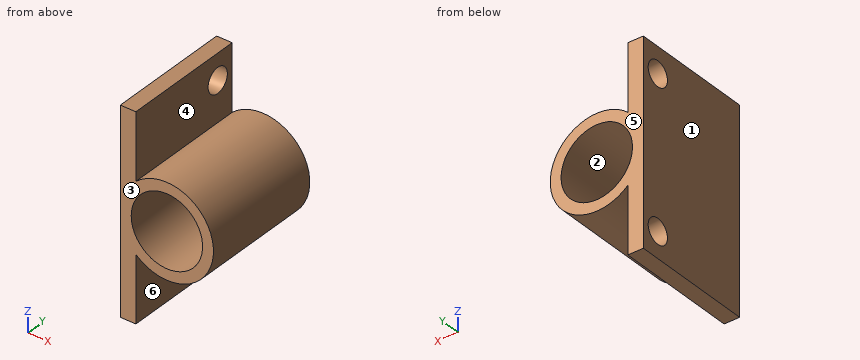
Autodesk Inventor part; units mm, degrees
ref_plane "YZ Plane" through (0, 0, 0) normal (1, 0, 0) x (0, 1, 0)
ref_plane "XZ Plane" through (0, 0, 0) normal (0, 1, 0) x (-1, 0, 0)
ref_plane "XY Plane" through (0, 0, 0) normal (0, 0, 1) x (1, 0, 0)
sketch "Sketch1" plane through (0, 0, 0) normal (0, 1, 0) x (-1, 0, 0)
  circle A0 centre (0, 0) radius 4.6
  line L0 (6, 13) -> (4, 13)
  line L1 (6, -13) -> (4, -13)
  arc A1 (4, 4.4721) -> (4, -4.4721) centre (0, 0) ccw
  line L2 (4, 13) -> (4, 4.4721)
  line L3 (4, -4.4721) -> (4, -13)
  line L4 (6, 13) -> (6, -13)
  dimension "d0" = 9.2
  dimension "d2" = 26
  dimension "d3" = 2
extrude "Extrusion1" add sketch "Sketch1" along normal blind 16
sketch "Sketch2" plane through (-6, 0, -13) normal (-1, 0, 0) x (0, 0, 1)
  circle A0 centre (3.35, 13.6) radius 1.6
  circle A1 centre (22.65, 13.6) radius 1.6
  line L0 (8.5279, 16) -> (0, 16)
  line L1 (0, 16) -> (26, 16)
  point P0 (13, 0)
  dimension "d10" = 3.2
  dimension "d11" = 3.2
  dimension "d14" = 2.4
  dimension "d15" = 2.4
extrude "Extrusion2" cut sketch "Sketch2" against normal blind 16
properties part number "Support endStop v2"
Geometry: final body of the model. Coordinates: model frame, mm. Face numbers are marked on the shaded views. A direction names the side the tool comes from. Round coordinates to 2 decimals unless told otherwise and drop trailing zeros. Loops run counter-clockwise (first coordinate to the right, second up) from the corner with the lowest first, then second, coordinate; pieces in that order, holes last. Notation, with made-up numbers: M -35.75,20.5 L 5.25,20.5 A26 ccw 5.25,55.5 Z; hole C 16,-27.5 d9. An arc over 180 degrees is marked long. Put each result on its own line as item: value. Start each with the question number.
(1) Draft query along X for the marked faces 1, 2 and 3. Return one class per face: +X half, -X half, draft (parallel to the pull), parting line (faces both ways), or undercut.
(2) Contact query for flat-ended pins moving along their axis: pin 1 Ø6 at (x, y) = (-3, 12) entering from +Z; pin 2 Ø4.5 at (y, z) = (9, 7.5) entering from +X; pin 3 Ø2 at (x, y) = (-0.5, 10) entering from +Z; pin 4 Ø9.5 at (y, z) = (8, -9) entering from +X. Output: stop coordinate, or through.
(3) Section query A-A (y = 13.6). Return loops of the section in (x, z), then the cut area to 3 significant figures.
(4) Material intervals for line 1 along Y through (x, z) = (-4.8, -9.65); line 2 along Z through (x, y) = (-0.25, 5); line 3 along X through (y, z) = (5.75, 8.75), sorted ascending. Write a range as [from, to].
(5) Section query C-C (z = 0). Return loops of the section in (x, y).
(6) Section query D-D (y = 2.5). Return loops of the section in (x, z).
(7) Set-up query: the marked faces 4, 5 and 6. Return all of +Z, -Z, +X, -X, +Y, -Y with unobstructed straight access to the full face (end or side cutting, diameter ignored); none if empty.
(8) Section query B-B (x = 0). Return loops of the section in (y, z), then the cut area to 3 significant figures.
Findings below:
1. face 1: -X half
1. face 2: undercut
1. face 3: draft
2. pin 1: stops at z = 13
2. pin 2: stops at x = 2.9
2. pin 3: stops at z = 6
2. pin 4: stops at x = 4.24
3. outline: M -6,-13 L -4,-13 L -4,-11.25 L -6,-11.25 Z; M -6,-8.05 L -4,-8.05 L -4,-4.47 A6 ccw long -4,4.47 L -4,8.05 L -6,8.05 Z; M -6,11.25 L -4,11.25 L -4,13 L -6,13 Z; hole C 0,0 d9.2
3. area: 73.4 mm2
4. line 1: y = [0, 12], [15.2, 16]
4. line 2: z = [-5.99, -4.59], [4.59, 5.99]
4. line 3: x = [-6, -4]
5. outline: M -6,0 L -4.6,0 L -4.6,16 L -6,16 Z; M 4.6,0 L 6,0 L 6,16 L 4.6,16 Z
6. outline: M -6,-13 L -4,-13 L -4,-4.47 A6 ccw long -4,4.47 L -4,13 L -6,13 Z; hole C 0,0 d9.2
7. face 4: +Z, +Y, -Y
7. face 5: +Z, -Z, +X, -X, +Y
7. face 6: -Z, +Y, -Y
8. outline: M 0,-6 L 16,-6 L 16,-4.6 L 0,-4.6 Z; M 0,4.6 L 16,4.6 L 16,6 L 0,6 Z
8. area: 44.8 mm2
